Autodesk Inventor part; units mm, degrees
ref_plane "YZ Plane" through (0, 0, 0) normal (1, 0, 0) x (0, 1, 0)
ref_plane "XZ Plane" through (0, 0, 0) normal (0, 1, 0) x (-1, 0, 0)
ref_plane "XY Plane" through (0, 0, 0) normal (0, 0, 1) x (1, 0, 0)
sketch "Sketch1" plane through (0, 0, 0) normal (0, 1, 0) x (-1, 0, 0)
  circle A0 centre (0, 0) radius 24
  circle A1 centre (0, 0) radius 21.25 construction
  circle A2 centre (0, -21.25) radius 1.8
  circle A3 centre (18.403, -10.625) radius 1.8
  circle A4 centre (18.403, 10.625) radius 1.8
  circle A5 centre (0, 21.25) radius 1.8
  circle A6 centre (-18.403, 10.625) radius 1.8
  circle A7 centre (-18.403, -10.625) radius 1.8
  dimension "d9" = 42.5
  dimension "d7" = 48
  dimension "d11" = 3.6
  dimension "d22" = 360
extrude "Extrusion1" add sketch "Sketch1" along normal blind 3
sketch "Sketch2" plane through (0, 3, 0) normal (0, 1, 0) x (1, 0, 0)
  circle A0 centre (0, 0) radius 17.75
  dimension "d26" = 35.5
extrude "Extrusion3" add sketch "Sketch2" along normal blind 9.7
equation "\"d9\" = iciclesMountD"
equation "\"d7\" = iciclesBaseOuterD"
equation "\"d11\" = clearanceM6"
equation "\"d24\" = isiclesBaseThickness"
equation "\"d26\" = iciclesPlugD"
equation "\"d30\" = chairThickness - isiclesBaseThickness"
equation "\"moduleHeight\" = 96"
equation "\"moduleMountD\" = 6.8"
equation "\"moduleCornerR\" = 5"
equation "\"d4\" = moduleCornerR"
equation "\"d5\" = moduleMountD"
equation "\"d6\" = moduleMountD"
equation "\"d8\" = moduleMountD"
equation "\"d10\" = moduleMountD"
equation "\"moduleOpeningR\" = 25"
equation "\"d13\" = moduleOpeningR"
equation "\"thickness\" = 6"
equation "\"d15\" = thickness"
equation "\"d16\" = 0"
equation "\"iciclesMountD\" = 42.5"
equation "\"d17\" = iciclesMountD"
equation "\"clearanceM6\" = 3.6"
equation "\"d18\" = clearanceM6"
equation "\"d21\" = 360deg"
equation "\"d0\" = moduleHeight"
equation "\"iciclesBaseOuterD\" = 48"
equation "\"iciclesPlugD\" = 35.5"
equation "\"chairThickness\" = 12.7"
equation "\"isiclesBaseThickness\" = 3"
properties part number "Module_bottom_Icicles26"
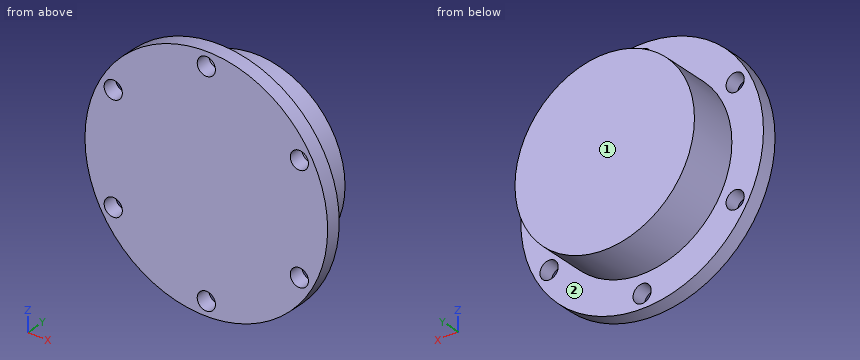
Geometry check sheet. Reference: the model listing, model coordinates, mm. Face numbers are marked on the shaded views. A direction names the side the tool comes from. Give positions to 0.01 mm unless a question says otherwise; leave off trailing zeros. Loops run counter-clockwise (first coordinate to the right, second up) from the corner with the lowest first, then second, coordinate; pieces in that order, holes last. Notation, with made-up numbers: M 30.5,79 L 42.5,79 A28 ccw 42.5,99 Z; hole C 41.25,-21 d1. An arc over 180 degrees is marked long. Answer as a JSON object with one key per item and string values. Group by question number.
Item 1: Gauge pin test, flat ends, axial feed: pin 1 (3 mm diameter, centred on x = -4.5, y = 2, fed in from -Z); pin 2 (3 mm diameter, centred on x = 0, z = -21.25, fed in from -Y); pin 3 (2 mm diameter, centred on x = 10, y = 7.5, fed in from -Z); pin 4 (6 mm diameter, centred on x = 0, z = 21.25, fed in from +Y). Record the tip position at first contact, or that the pin passes through.
Item 2: Sectioned sample at C-C on z = -21.25. Record the boundary of the cut face in (x, y), plus the area to 3 significant figures.
Item 3: Access from +Z, -Z, +X, -X, +Y, -Y to the whole of each face (thin tool, end or side, straight path). Record for the marked faces 1 and 2.
Item 4: Material ranges on L1, parallel to Z at x = 0, y = 2.2; L2, parallel to Y at x = -10, z = 20.5; L3, parallel to X at y = 8, z = 0, recorded low to high.
Item 5: Sectioned sample at A-A on x = 0. Record the boundary of the cut face in (y, z), plus the area to 3 significant figures.
Item 6: Sectioned sample at B-B on z = 0. Record the boundary of the cut face in (x, y), plus the area to 3 significant figures.
Item 7: Sectioned sample at D-D on y = 9.25. Record the boundary of the cut face in (x, z).
Findings below:
{
 "1": {"pin 1": "z = -23.81", "pin 2": "through", "pin 3": "z = -15.3", "pin 4": "y = 3"},
 "2": {"outline": "M -11.16,0 L -1.8,0 L -1.8,3 L -11.16,3 Z; M 1.8,0 L 11.16,0 L 11.16,3 L 1.8,3 Z", "area": "56.1 mm2"},
 "3": {"face 1": "+Z, -Z, +X, -X, +Y", "face 2": "+Y"},
 "4": {"L1": "-24 to -23.05, -19.45 to 19.45, 23.05 to 24", "L2": "0 to 3", "L3": "-17.75 to 17.75"},
 "5": {"outline": "M 0,-24 L 3,-24 L 3,-23.05 L 0,-23.05 Z; M 0,-19.45 L 3,-19.45 L 3,-17.75 L 12.7,-17.75 L 12.7,17.75 L 3,17.75 L 3,19.45 L 0,19.45 Z; M 0,23.05 L 3,23.05 L 3,24 L 0,24 Z", "area": "467 mm2"},
 "6": {"outline": "M -24,0 L 24,0 L 24,3 L 17.75,3 L 17.75,12.7 L -17.75,12.7 L -17.75,3 L -24,3 Z", "area": "488 mm2"},
 "7": {"outline": "C 0,0 d35.5"}
}
